Study the drawing (mm; zero at the part's minimum x, y, z) and answer. A direction names the side the tool comes from. Coordinates: 2 decimals unless noted, no trailing zeros. Loops run counter-clockwise (first coordinate to the right, second up) from the corner with the lowest first, then second, coordinate; pieces in that order, holes last. Notation, with made-up numbers: (5, -32.75) - (26, -32.75) arc R21 ccw to (26, -16.75) - close; hole circle Ø4 at (-13.5, 13.25). An arc over 180 degrees is marked (long way). Use CSV: the item, a comma, the result in double quotes.
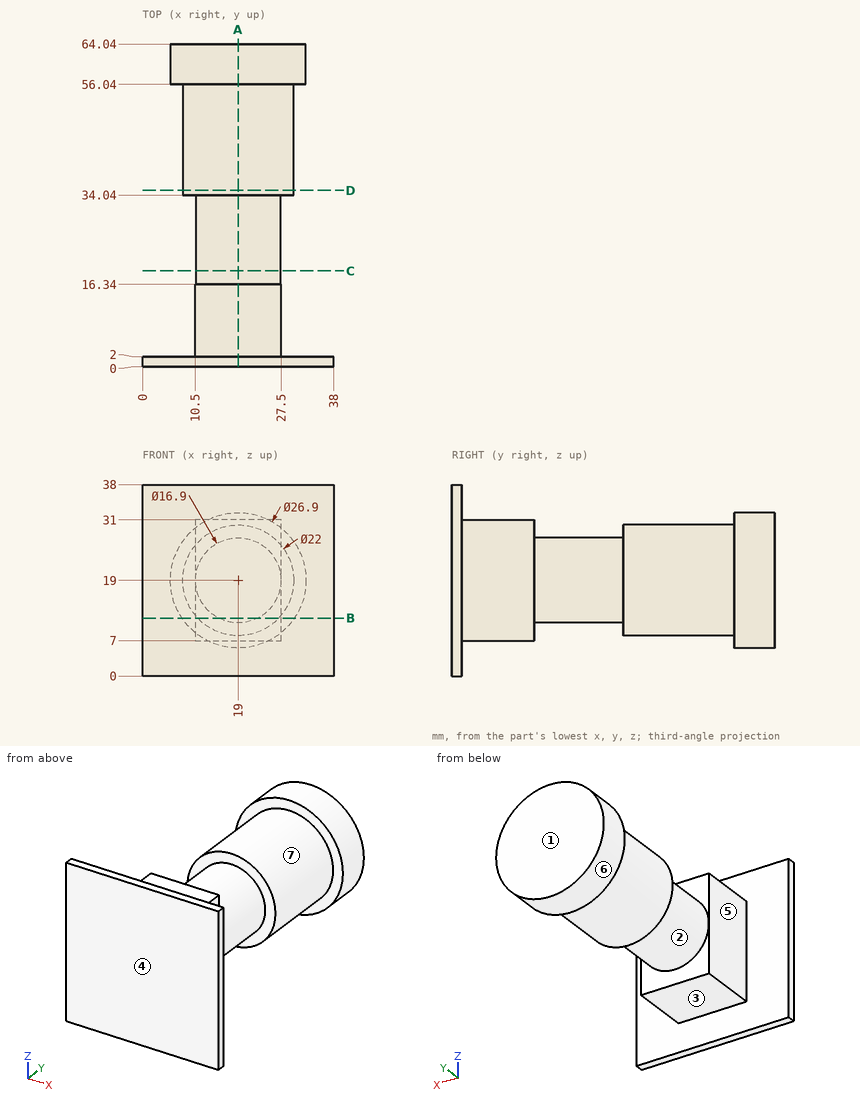
Q1. The part is cut by section B-B on z = 11.5. Determine the outline of the cut face in (x, y).
Reported:
outline,"(0, 0) - (38, 0) - (38, 2) - (27.5, 2) - (27.5, 16.34) - (22.89, 16.34) - (22.89, 34.04) - (27.05, 34.04) - (27.05, 56.04) - (30.16, 56.04) - (30.16, 64.04) - (7.84, 64.04) - (7.84, 56.04) - (10.95, 56.04) - (10.95, 34.04) - (15.11, 34.04) - (15.11, 16.34) - (10.5, 16.34) - (10.5, 2) - (0, 2) - close"
Q2. For a pull along Y with two mould halves and no side action, classify the marked faces 1, 2, 3 and 4 as +Y half, -Y half, draft (parallel to the pull), parting line (faces both ways), or undercut.
Reported:
face 1,"+Y half"
face 2,"undercut"
face 3,"undercut"
face 4,"-Y half"
Q3. The part is cut by section A-A on x = 19. Determine the outline of the cut face in (y, z), and give its area (3 significant figures).
Reported:
outline,"(0, 0) - (2, 0) - (2, 7) - (16.34, 7) - (16.34, 10.55) - (34.04, 10.55) - (34.04, 8) - (56.04, 8) - (56.04, 5.55) - (64.04, 5.55) - (64.04, 32.45) - (56.04, 32.45) - (56.04, 30) - (34.04, 30) - (34.04, 27.45) - (16.34, 27.45) - (16.34, 31) - (2, 31) - (2, 38) - (0, 38) - close"
area,"1,420 mm²"
Q4. Find the intervals of material crossed by probe 1 along Y at (x, z) = (14.5, 11.5); probe 2 along Y at (x, z) = (32, 21); probe 3 along Z at (x, y) = (19, 42), in increasing order. Write a range as [from, to].
Reported:
probe 1,"y = [0, 16.34], [34.04, 64.04]"
probe 2,"y = [0, 2], [56.04, 64.04]"
probe 3,"z = [8, 30]"
Q5. The part is cut by section C-C on y = 19. Determine the outline of the cut face in (x, z), and give its area (3 significant figures).
Reported:
outline,"circle Ø16.9 at (19, 19)"
area,"224 mm²"
Q6. The part is cut by section D-D on y = 35. Determine the outline of the cut face in (x, z).
Reported:
outline,"circle Ø22 at (19, 19)"
Q7. Given P1, Ø8, axis at x = 28, y = 29.5, coming from the +Z side; P2, Ø4.5, axis at x = 19.5, y = 12.5, coming from the +Z side; P3, Ø1.5, axis at x = 9, y = 35.5, coming from the -Z side, each flat-ended and moving along its own axis, determine where each tip first touches the part or whether it passes through.
Reported:
P1,"stops at z = 25.81"
P2,"stops at z = 31"
P3,"stops at z = 13.05"
Q8. A tool of negligible diameter and unlimited length cuts with its end or side. For the marked faces 5, 6 and 7, from which of +Z, -Z, +X, -X, +Y, -Y can it reach the whole face along a straight path? Write none if from no direction.
Reported:
face 5,"+Z, -Z, -X"
face 6,"+Y"
face 7,"none"
